Drawing for the job (mm, zero at the part's lowest x, y, z). A direction names the side the tool comes from. Coordinates: 2 decimals unless noted, no trailing zeros. Write each loop counter-clockwise with the first axis right and the second up, starting at its lowest first coordinate (ties: lowest second). Pieces come first, ordered by that corner, then holes. Notation, with made-up numbers: (14.25, 85) - (18.25, 85) arc R21 ccw to (18.25, 100) - close; hole circle Ø1 at (-1, 86.25). An arc over 180 degrees is marked (long way). Write each question's results on one line, items separated by ' | '.
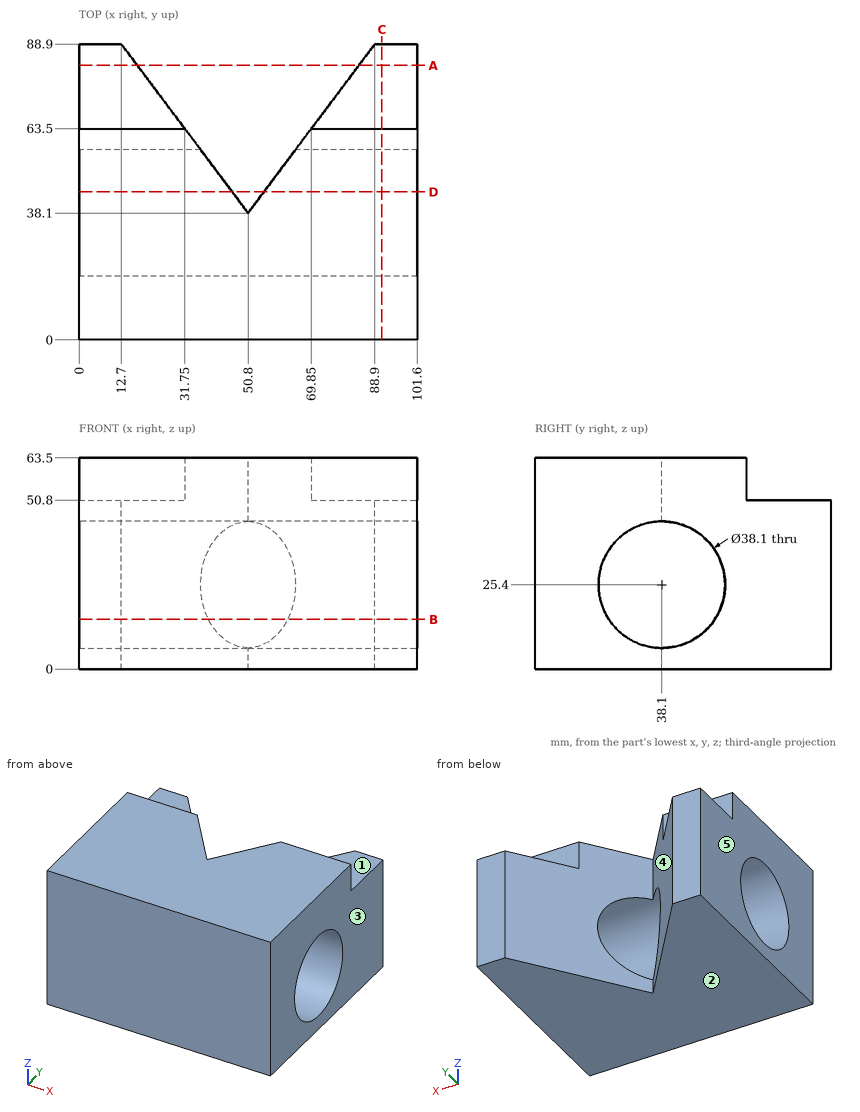
(1) Saw through at C-C on x = 91. Write the cut outline in (y, z).
Return value:
outline: (0, 0) - (88.9, 0) - (88.9, 50.8) - (63.5, 50.8) - (63.5, 63.5) - (0, 63.5) - close; hole circle Ø38.1 at (38.1, 25.4)
(2) Saw through at D-D on y = 44.5. Write the cut outline in (x, z).
Return value:
outline: (0, 0) - (46, 0) - (46, 7.46) - (0, 7.46) - close; (0, 43.34) - (46, 43.34) - (46, 63.5) - (0, 63.5) - close; (55.6, 0) - (101.6, 0) - (101.6, 7.46) - (55.6, 7.46) - close; (55.6, 43.34) - (101.6, 43.34) - (101.6, 63.5) - (55.6, 63.5) - close
(3) Flat gauge pins, fed straight in: P1, Ø10, axis at x = 12.5, z = 58.5, coming from the +Y side; P2, Ø20.5, axis at x = 84.5, y = 78, coming from the +Z side; P3, Ø5, axis at x = 22, z = 23, coming from the +Y side. Where does each tip first touch, or does it go through?
Return value:
P1: stops at y = 63.5 | P2: stops at z = 50.8 | P3: stops at y = 79.83
(4) 3-axis set-ups, long thin cutter, end or side, ignore diameter. For the marked faces 1 and 2: which of +Z, -Z, +X, -X, +Y, -Y reach the whole face in a straight line?
Return value:
face 1: +Z, +X, -X, +Y | face 2: -Z, +X, -X, +Y, -Y
(5) Wall check: line 1 (Z direction, x = 61, y = 38); line 2 (Y direction, x = 20, z = 22.5); line 3 (Z direction, x = 96, y = 65.5). Give the ranges that are in metal, low to high. Write a range as from..to.
Return value:
line 1: z = 0..6.35, 44.45..63.5 | line 2: y = 0..19.27, 56.93..79.17 | line 3: z = 0..50.8
(6) Two-plate mould, pull along X, no slides. Class the marked faces 3, 4 and 5: released by +X, released by -X, zero draft, split by the parting line, or undercut.
Return value:
face 3: released by +X | face 4: undercut | face 5: released by -X
(7) Saw through at A-A on y = 82.5. Write the cut outline in (x, z).
Return value:
outline: (0, 0) - (17.5, 0) - (17.5, 50.8) - (0, 50.8) - close; (84.1, 0) - (101.6, 0) - (101.6, 50.8) - (84.1, 50.8) - close
(8) Saw through at B-B on z = 15. Write the cut outline in (x, y), then the cut area to 3 significant figures.
Return value:
outline: (0, 0) - (101.6, 0) - (101.6, 22.14) - (0, 22.14) - close; (0, 54.06) - (38.83, 54.06) - (12.7, 88.9) - (0, 88.9) - close; (62.77, 54.06) - (101.6, 54.06) - (101.6, 88.9) - (88.9, 88.9) - close | area: 4,040 mm^2
